Work out the finished part from the listing and answer in its coordinate system (mm). Face numbers are marked on the shaded views. A direction names the side the tool comes from. Coordinates: 2 decimals unless noted, no trailing zeros. Loops run counter-clockwise (first coordinate to the right, second up) from the corner with the lowest first, then second, coordinate; pieces in that order, holes last.
```python
from build123d import *

# Parameters (mm, degrees)
SKETCH1_R           = 45
BOSS_EXTRUDE1_DEPTH = 10
SKETCH2_R           = 5
BOSS_EXTRUDE2_DEPTH = 10
SKETCH3_R           = 10
BOSS_EXTRUDE3_DEPTH = 60
BOSS_EXTRUDE4_START = 15
SKETCH4_R           = 45
BOSS_EXTRUDE4_DEPTH = 15
CUT_EXTRUDE1_START  = -2.5
SKETCH5_R           = 45
SKETCH5_R_2         = 42.5
CUT_EXTRUDE1_DEPTH  = 10


with BuildPart() as part:
    # Sketch1 → Boss-Extrude1 (new body)
    with BuildSketch(Plane.XY):
        Circle(SKETCH1_R)
    extrude(amount=BOSS_EXTRUDE1_DEPTH)

    # Sketch2 → Boss-Extrude2 (add)
    with BuildSketch(Plane.XY.offset(20)):
        with Locations((-40, 0)):
            Circle(SKETCH2_R)
    extrude(amount=-BOSS_EXTRUDE2_DEPTH)

    # Sketch3 → Boss-Extrude3 (add)
    with BuildSketch(Plane(origin=(0, 0, 0), x_dir=(-1, 0, 0), z_dir=(0, 0, -1))):
        Circle(SKETCH3_R)
    extrude(amount=BOSS_EXTRUDE3_DEPTH)

    # Sketch4 → Boss-Extrude4 (add)
    with BuildSketch(Plane(origin=(0, 0, -60), x_dir=(-1, 0, 0), z_dir=(0, 0, -1)).offset(BOSS_EXTRUDE4_START)):
        Circle(SKETCH4_R)
    extrude(amount=-BOSS_EXTRUDE4_DEPTH)

    # Sketch5 → Cut-Extrude1 (cut)
    with BuildSketch(Plane(origin=(0, 0, -75), x_dir=(-1, 0, 0), z_dir=(0, 0, -1)).offset(CUT_EXTRUDE1_START)):
        Circle(SKETCH5_R)
        Circle(SKETCH5_R_2, mode=Mode.SUBTRACT)
    extrude(amount=-CUT_EXTRUDE1_DEPTH, mode=Mode.SUBTRACT)


solid = part.part
```
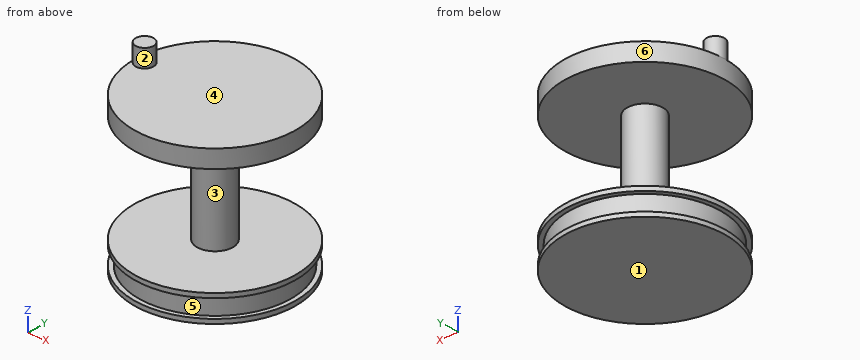
1. Each of these flat-tipped pins is pushed along its axis until it touches: P1, Ø2, axis at y = 8.5, z = -6, coming from the -X side; P2, Ø5, axis at x = 13.5, y = 6, coming from the +Z side; P3, Ø1, axis at y = -27, z = 1, coming from the +X side. Where does it stop, or does it pass through?
2. A cutting plane is placed at D-D, the plane x = 0. Give the vertices of the cut face in (y, z), then the cut area to 3 significant figures.
3. A cutting plane is placed at C-C, the plane z = -39. Give the vertices of the cut face in (x, y).
4. Determine the mould class of the marked faces 4, 5 and 6 for opening direction Z: released by +Z, released by -Z, zero draft, split by the parting line, or undercut.
5. For the marked faces 1, 2 and 3, determine the directions among +Z, -Z, +X, -X, +Y, -Y from which every point of the face is accessible in a straight line to the end or side of a thin tool.
6. A cutting plane is placed at A-A, the plane x = -40. Give the vertices of the cut face in (y, z), then the cut area to 3 significant figures.
7. Straight lines are drawn through the part: probe 1 along Z at (x, y) = (-11, 2); probe 2 along Z at (x, y) = (4.5, 3.5); probe 3 along Y at (x, z) = (0, -57.5). For each, find the intervals that lie inside material, in ascending order.
8. A cutting plane is placed at B-B, the plane y = -33. Give the vertices of the cut face in (x, z), then the cut area to 3 significant figures.
Answers below:
1. P1: stops at x = -6.61
1. P2: stops at z = 10
1. P3: stops at x = 36.37
2. outline: (-45, -75) - (45, -75) - (45, -72.5) - (42.5, -72.5) - (42.5, -62.5) - (45, -62.5) - (45, -60) - (10, -60) - (10, 0) - (45, 0) - (45, 10) - (-45, 10) - (-45, 0) - (-10, 0) - (-10, -60) - (-45, -60) - (-45, -62.5) - (-42.5, -62.5) - (-42.5, -72.5) - (-45, -72.5) - close
2. area: 3,400 mm2
3. outline: circle Ø20 at (0, 0)
4. face 4: released by +Z
4. face 5: undercut
4. face 6: zero draft
5. face 1: -Z, +X, -X, +Y, -Y
5. face 2: +Z
5. face 3: none
6. outline: (-20.62, -75) - (20.62, -75) - (20.62, -72.5) - (14.36, -72.5) - (14.36, -62.5) - (20.62, -62.5) - (20.62, -60) - (-20.62, -60) - (-20.62, -62.5) - (-14.36, -62.5) - (-14.36, -72.5) - (-20.62, -72.5) - close; (-20.62, 0) - (20.62, 0) - (20.62, 10) - (5, 10) - (5, 20) - (-5, 20) - (-5, 10) - (-20.62, 10) - close
6. area: 1,010 mm2
7. probe 1: z = -75 to -60, 0 to 10
7. probe 2: z = -75 to 10
7. probe 3: y = -10 to 10
8. outline: (-30.59, -75) - (30.59, -75) - (30.59, -72.5) - (26.78, -72.5) - (26.78, -62.5) - (30.59, -62.5) - (30.59, -60) - (-30.59, -60) - (-30.59, -62.5) - (-26.78, -62.5) - (-26.78, -72.5) - (-30.59, -72.5) - close; (-30.59, 0) - (30.59, 0) - (30.59, 10) - (-30.59, 10) - close
8. area: 1,450 mm2
